```python
from build123d import *

# Parameters (mm, degrees)
BOSS_EXTRUDE1_DEPTH = 102.8
CUT_EXTRUDE1_DEPTH  = 103.8
CUT_EXTRUDE2_DEPTH  = 103.8
CUT_EXTRUDE3_REACH  = 89.934
SKETCH5_R           = 1.65
CUT_EXTRUDE4_START  = -5
CUT_EXTRUDE4_DEPTH  = 83.934228689
SKETCH7_R           = 0.95
CUT_EXTRUDE5_DEPTH  = 103.8


with BuildPart() as part:
    # Sketch1 → Boss-Extrude1 (new body)
    with BuildSketch(Plane.XY):
        with BuildLine():
            Line((0, 59), (0, 43))
            ThreePointArc((0, 43), (-43, 0), (0, -43))
            Line((0, -43), (0, -59))
            ThreePointArc((0, -59), (-59, 0), (0, 59))
        make_face()
    extrude(amount=BOSS_EXTRUDE1_DEPTH)

    # Sketch3 → Cut-Extrude1 (cut, through all)
    with BuildSketch(Plane.XY.offset(102.8)):
        Polygon((0, 0), (0, 90), (-70.757321084, 90), (-38, 0), align=None)
    extrude(amount=-CUT_EXTRUDE1_DEPTH, mode=Mode.SUBTRACT)

    # Sketch4 → Cut-Extrude2 (cut, through all)
    with BuildSketch(Plane.XY.offset(102.8)):
        Polygon((0, -59), (-29.014256172, -51.372881356), (-31.019233948, -59), align=None)
    extrude(amount=-CUT_EXTRUDE2_DEPTH, mode=Mode.SUBTRACT)

    # Sketch5 → Cut-Extrude3 (cut, up to next)
    with BuildSketch(Plane(origin=(-14.507128086, -55.186440678, 0), x_dir=(0.967141872, -0.254237288, 0), z_dir=(-0.254237288, -0.967141872, 0)), mode=Mode.PRIVATE) as cut_extrude3_sk1:
        with Locations((-1, 20)):
            Circle(SKETCH5_R)
    cut_extrude3_tool1 = extrude(cut_extrude3_sk1.sketch, amount=-CUT_EXTRUDE3_REACH, mode=Mode.PRIVATE) & part.part
    add(cut_extrude3_tool1.solids().sort_by_distance((-15.47427, -54.932203, 20))[0], mode=Mode.SUBTRACT)
    # Sketch5 → Cut-Extrude3 (cut, up to next)
    with BuildSketch(Plane(origin=(-14.507128086, -55.186440678, 0), x_dir=(0.967141872, -0.254237288, 0), z_dir=(-0.254237288, -0.967141872, 0)), mode=Mode.PRIVATE) as cut_extrude3_sk2:
        with Locations((-1, 10)):
            Circle(SKETCH5_R)
    cut_extrude3_tool2 = extrude(cut_extrude3_sk2.sketch, amount=-CUT_EXTRUDE3_REACH, mode=Mode.PRIVATE) & part.part
    add(cut_extrude3_tool2.solids().sort_by_distance((-15.47427, -54.932203, 10))[0], mode=Mode.SUBTRACT)
    # Sketch5 → Cut-Extrude3 (cut, up to next)
    with BuildSketch(Plane(origin=(-14.507128086, -55.186440678, 0), x_dir=(0.967141872, -0.254237288, 0), z_dir=(-0.254237288, -0.967141872, 0)), mode=Mode.PRIVATE) as cut_extrude3_sk3:
        with Locations((-1, 92.8)):
            Circle(SKETCH5_R)
    cut_extrude3_tool3 = extrude(cut_extrude3_sk3.sketch, amount=-CUT_EXTRUDE3_REACH, mode=Mode.PRIVATE) & part.part
    add(cut_extrude3_tool3.solids().sort_by_distance((-15.47427, -54.932203, 92.8))[0], mode=Mode.SUBTRACT)
    # Sketch5 → Cut-Extrude3 (cut, up to next)
    with BuildSketch(Plane(origin=(-14.507128086, -55.186440678, 0), x_dir=(0.967141872, -0.254237288, 0), z_dir=(-0.254237288, -0.967141872, 0)), mode=Mode.PRIVATE) as cut_extrude3_sk4:
        with Locations((-1, 82.8)):
            Circle(SKETCH5_R)
    cut_extrude3_tool4 = extrude(cut_extrude3_sk4.sketch, amount=-CUT_EXTRUDE3_REACH, mode=Mode.PRIVATE) & part.part
    add(cut_extrude3_tool4.solids().sort_by_distance((-15.47427, -54.932203, 82.8))[0], mode=Mode.SUBTRACT)
    # Sketch5 → Cut-Extrude3 (cut, up to next)
    with BuildSketch(Plane(origin=(-14.507128086, -55.186440678, 0), x_dir=(0.967141872, -0.254237288, 0), z_dir=(-0.254237288, -0.967141872, 0)), mode=Mode.PRIVATE) as cut_extrude3_sk5:
        with Locations((7, 20)):
            Circle(SKETCH5_R)
    cut_extrude3_tool5 = extrude(cut_extrude3_sk5.sketch, amount=-CUT_EXTRUDE3_REACH, mode=Mode.PRIVATE) & part.part
    add(cut_extrude3_tool5.solids().sort_by_distance((-7.737135, -56.966102, 20))[0], mode=Mode.SUBTRACT)
    # Sketch5 → Cut-Extrude3 (cut, up to next)
    with BuildSketch(Plane(origin=(-14.507128086, -55.186440678, 0), x_dir=(0.967141872, -0.254237288, 0), z_dir=(-0.254237288, -0.967141872, 0)), mode=Mode.PRIVATE) as cut_extrude3_sk6:
        with Locations((7, 10)):
            Circle(SKETCH5_R)
    cut_extrude3_tool6 = extrude(cut_extrude3_sk6.sketch, amount=-CUT_EXTRUDE3_REACH, mode=Mode.PRIVATE) & part.part
    add(cut_extrude3_tool6.solids().sort_by_distance((-7.737135, -56.966102, 10))[0], mode=Mode.SUBTRACT)
    # Sketch5 → Cut-Extrude3 (cut, up to next)
    with BuildSketch(Plane(origin=(-14.507128086, -55.186440678, 0), x_dir=(0.967141872, -0.254237288, 0), z_dir=(-0.254237288, -0.967141872, 0)), mode=Mode.PRIVATE) as cut_extrude3_sk7:
        with Locations((7, 92.8)):
            Circle(SKETCH5_R)
    cut_extrude3_tool7 = extrude(cut_extrude3_sk7.sketch, amount=-CUT_EXTRUDE3_REACH, mode=Mode.PRIVATE) & part.part
    add(cut_extrude3_tool7.solids().sort_by_distance((-7.737135, -56.966102, 92.8))[0], mode=Mode.SUBTRACT)
    # Sketch5 → Cut-Extrude3 (cut, up to next)
    with BuildSketch(Plane(origin=(-14.507128086, -55.186440678, 0), x_dir=(0.967141872, -0.254237288, 0), z_dir=(-0.254237288, -0.967141872, 0)), mode=Mode.PRIVATE) as cut_extrude3_sk8:
        with Locations((7, 82.8)):
            Circle(SKETCH5_R)
    cut_extrude3_tool8 = extrude(cut_extrude3_sk8.sketch, amount=-CUT_EXTRUDE3_REACH, mode=Mode.PRIVATE) & part.part
    add(cut_extrude3_tool8.solids().sort_by_distance((-7.737135, -56.966102, 82.8))[0], mode=Mode.SUBTRACT)

    # Sketch6 → Cut-Extrude4 (cut, through all)
    with BuildSketch(Plane(origin=(-14.507128086, -55.186440678, 0), x_dir=(0.967141872, -0.254237288, 0), z_dir=(-0.254237288, -0.967141872, 0)).offset(CUT_EXTRUDE4_START)):
        Polygon((7, 95.972596752), (4.252450617, 94.386298376), (4.252450617, 91.213701624), (7, 89.627403248), (9.747549383, 91.213701624), (9.747549383, 94.386298376), align=None)
        Polygon((1.680535984, 91.097631011), (1.814562783, 94.270227763), (-0.865973201, 95.972596752), (-3.680535984, 94.502368989), (-3.814562783, 91.329772237), (-1.134026799, 89.627403248), align=None)
        Polygon((1.680535984, 81.097631011), (1.814562783, 84.270227763), (-0.865973201, 85.972596752), (-3.680535984, 84.502368989), (-3.814562783, 81.329772237), (-1.134026799, 79.627403248), align=None)
        Polygon((1.680535984, 21.702368989), (-1.134026799, 23.172596752), (-3.814562783, 21.470227763), (-3.680535984, 18.297631011), (-0.865973201, 16.827403248), (1.814562783, 18.529772237), align=None)
        Polygon((1.680535984, 11.702368989), (-1.134026799, 13.172596752), (-3.814562783, 11.470227763), (-3.680535984, 8.297631011), (-0.865973201, 6.827403248), (1.814562783, 8.529772237), align=None)
        Polygon((7, 85.972596752), (4.252450617, 84.386298376), (4.252450617, 81.213701624), (7, 79.627403248), (9.747549383, 81.213701624), (9.747549383, 84.386298376), align=None)
        Polygon((7, 23.172596752), (4.252450617, 21.586298376), (4.252450617, 18.413701624), (7, 16.827403248), (9.747549383, 18.413701624), (9.747549383, 21.586298376), align=None)
        Polygon((7, 13.172596752), (4.252450617, 11.586298376), (4.252450617, 8.413701624), (7, 6.827403248), (9.747549383, 8.413701624), (9.747549383, 11.586298376), align=None)
    extrude(amount=-CUT_EXTRUDE4_DEPTH, mode=Mode.SUBTRACT)

    # Sketch7 → Cut-Extrude5 (cut, through all)
    with BuildSketch(Plane(origin=(0, 0, 0), x_dir=(-1, 0, 0), z_dir=(0, 0, -1))):
        with Locations((24, -46)):
            Circle(SKETCH7_R)
        with Locations((51, -8)):
            Circle(SKETCH7_R)
    extrude(amount=-CUT_EXTRUDE5_DEPTH, mode=Mode.SUBTRACT)


solid = part.part
```
Input: part model. Units: mm. Frame: model coordinates. A direction names the side the tool comes from. Round coordinates to 2 decimals unless told otherwise and drop trailing zeros. Write each loop counter-clockwise with the first axis right and the second up, starting at its lowest first coordinate (ties: lowest second). Pieces come first, ordered by that corner, then holes. Notation, with made-up numbers: (-27, 20) -> (2, 20) arc R13 cw to (2, 39) -> close; hole circle Ø10 at (-17.5, -7.5). An arc over 180 degrees is marked (long way). Answer as CSV lines item,"result".
1. Contact query for flat-ended pins moving along their axis: P1, Ø3, axis at x = -30, z = 21.5, coming from the -Y side; P2, Ø12, axis at y = -14.5, z = 59, coming from the +X side; P3, Ø8, axis at y = -26, z = 19, coming from the -X side. Output: stop coordinate, or through.
Geometry says:
P1,"stops at y = -51.51"
P2,"stops at x = -37.8"
P3,"stops at x = -54.74"
2. Mould query, pull axis X, two halves, no side actions, for faces 1 (the cylindrical face through (-57.11, -14.82, 50.68)), 2 (the cylindrical face through (-16.114, -52.215, 8.996)), 3 (the cylindrical face through (-34.19, -26.08, 50.68)). Classes: +X half, -X half, draft (parallel to the pull), parting line (faces both ways), or undercut.
Geometry says:
face 1,"-X half"
face 2,"undercut"
face 3,"+X half"
3. Reachability of faces 4 (the flat face through (-7.68, -51.81, 18.63)), 5 (the flat face through (-2.53, -47.97, 82.78)) from +Z, -Z, +X, -X, +Y, -Y: full face, straight path, thin tool, end or side. Return the list, or none.
Geometry says:
face 4,"none"
face 5,"+Y"
4. Section C-C (x = -44.5). Return the cut outline in (y, z).
Geometry says:
outline,"(-38.74, 0) -> (17.86, 0) -> (17.86, 102.8) -> (-38.74, 102.8) -> close"
5. Section B-B (y = 19.5). Return the cut outline in (x, z).
Geometry says:
outline,"(-55.68, 0) -> (-45.1, 0) -> (-45.1, 102.8) -> (-55.68, 102.8) -> close"
6. Ray query, L1, parallel to Y at x = -51, z = 76.5; L2, parallel to Y at x = -24, z = 24; L3, parallel to X at y = -46, z = 72.5. Return the intervals inside material, ascending. Write a range as [from, to].
Geometry says:
L1,"y = [-29.66, -8.95], [-7.05, 29.66]"
L2,"y = [-52.69, -46.95], [-45.05, -35.68]"
L3,"x = [-36.95, -24.95], [-23.05, 0]"
7. Section A-A (z = 64). Return the cut outline in (x, y).
Geometry says:
outline,"(-49.62, 31.92) arc R59 ccw to (-29.01, -51.37) -> (0, -59) -> (0, -43) arc R43 cw to (-41.75, 10.3) -> close; hole circle Ø1.9 at (-51, -8); hole circle Ø1.9 at (-24, -46)"
